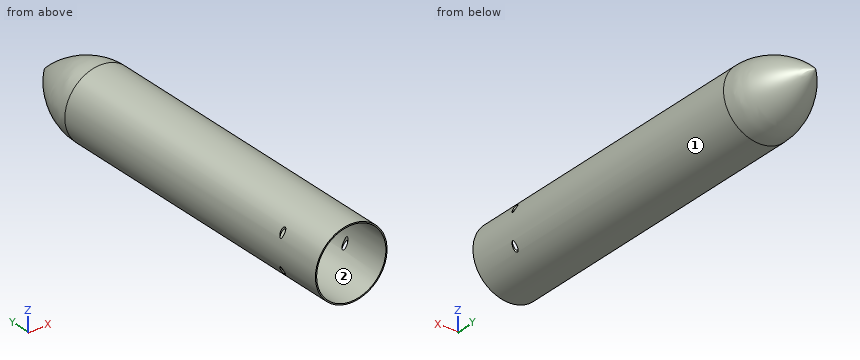
```python
from build123d import *

# Parameters (mm, degrees)
SKETCH2_R          = 10
CUT_EXTRUDE1_DEPTH = 151.0000001


with BuildPart() as part:
    # Sketch1 → Revolve1 (revolve)
    with BuildSketch(Plane.XY):
        with BuildLine():
            Line((-150, 0), (-150, 1340))
            add(Edge.make_bspline(
                [(0, 1640), (-150, 1490), (-150, 1340)],
                knots=[0, 0, 0, 1, 1, 1], degree=2))
            Line((0, 1640), (0, 1632.952723956))
            Line((0, 1632.952723956), (-5, 1627.803149448))
            add(Edge.make_bspline(
                [(-5, 1627.803149448), (-57.694245938, 1573.511585517), (-112.347233502, 1483.42653426), (-145.016403602, 1393.670587787), (-145, 1340)],
                knots=[0.029045994, 0.029045994, 0.029045994, 0.393153746, 0.635892248, 1, 1, 1], degree=2))
            Line((-145, 1340), (-145, 5))
            Line((-145, 5), (-145, 0))
            Line((-145, 0), (-150, 0))
        make_face()
    revolve(axis=Axis((0, 0, 0), (0, 1, 0)))

    # Sketch2 → Cut-Extrude1 (cut, symmetric)
    with BuildSketch(Plane.XY):
        with Locations((130, 200)):
            Circle(SKETCH2_R)
    cut_extrude1 = extrude(amount=CUT_EXTRUDE1_DEPTH, both=True, mode=Mode.SUBTRACT)

    # Mirror1: Cut-Extrude1 across plane
    add(cut_extrude1.mirror(Plane(origin=(0, 0, 0), x_dir=(0, 0, 1), z_dir=(1, 0, 0))), mode=Mode.SUBTRACT)


solid = part.part
```
Here's how the part is built. I have some questions about the finished solid (model axes, mm). Face numbers are marked on the shaded views. Coordinates: 2 decimals unless noted, no trailing zeros. Loops run counter-clockwise (first coordinate to the right, second up) from the corner with the lowest first, then second, coordinate; pieces in that order, holes last. Notation, with made-up numbers: (25, 43) - (48, 43) arc R5 ccw to (48, 51) - close; hole circle Ø3 at (61, 17.5). An arc over 180 degrees is marked (long way). Answer as CSV lines item,"result".
Q1. If I drill on L1, parallel to Z at x = 0, y = 598; L2, parallel to Z at x = -7, y = 676.5; L3, parallel to X at y = 531, z = 37.5, over which ranges is the centre line in solid material (lowest first)? Write a range as [from, to].
Response:
L1,"[-150, -145], [145, 150]"
L2,"[-149.84, -144.83], [144.83, 149.84]"
L3,"[-145.24, -140.07], [140.07, 145.24]"
Q2. If we section it at A-A, the plane y = 1120: Write out the boundary of the cut face in (x, z).
Response:
outline,"circle Ø300 at (0, 0); hole circle Ø290 at (0, 0)"
Q3. We'd pull the mould along Z, two halves only. Please class the marked faces 1 and 2: pulls with the +Z half, pulls with the -Z half, needs draft (parallel to the pull), parting line crosses it, or undercut.
Response:
face 1,"parting line crosses it"
face 2,"undercut"
Q4. For pin 1 (12 mm diameter, centred on x = -51.5, y = 628, fed in from +Z); pin 2 (1.5 mm diameter, centred on y = 801, z = -80.5, fed in from -X); pin 3 (4 mm diameter, centred on x = -112.5, z = -8.5, fed in from +Y), each with a flat end and sliding along its axis, tell me the tip position at first contact or that it passes through.
Response:
pin 1,"z = 142.93"
pin 2,"x = -127.04"
pin 3,"y = 1493.32"
